Geometry: final body of the model. Coordinates: model frame, mm. A direction names the side the tool comes from. Coordinates: 2 decimals unless noted, no trailing zeros. Order: outer loops, then holes, each group sorted by start corner. A loop starts at its lowest first (then second) coordinate and runs counter-clockwise, first axis right, second up. Notation, with made-up numbers: (43, 36) -> (51, 36) arc R24 cw to (51, 48) -> close; hole circle Ø8 at (55.5, 31.5). An arc over 180 degrees is marked (long way). Use one line per item in the form item = value.
```python
from build123d import *

# Parameters (mm, degrees)
SKETCH1_W           = 33
SKETCH1_H           = 8
SKETCH1_R           = 1.55
BOSS_EXTRUDE1_DEPTH = 4
SKETCH3_W           = 8
SKETCH3_H           = 8
BOSS_EXTRUDE2_DEPTH = 5.5
FILLET1_R           = 2


with BuildPart() as part:
    # Sketch1 → Boss-Extrude1 (new body)
    with BuildSketch(Plane(origin=(0, 0, 0), x_dir=(1, 0, 0), z_dir=(0, 1, 0))):
        with Locations((0.21875, 2.328125)):
            Rectangle(SKETCH1_W, SKETCH1_H)
        with Locations(Location((12.71875, 2.328125, 0), (0, 0, 270))):
            Circle(SKETCH1_R, mode=Mode.SUBTRACT)
    extrude(amount=BOSS_EXTRUDE1_DEPTH)

    # Sketch3 → Boss-Extrude2 (add)
    with BuildSketch(Plane.XZ):
        with Locations((-12.28125, -2.328125)):
            Rectangle(SKETCH3_W, SKETCH3_H)
    extrude(amount=BOSS_EXTRUDE2_DEPTH)

    # Fillet1
    fillet1_edges = [part.edges().sort_by_distance(p)[0] for p in [
        (-16.28125, -5.5, -2.328125),
        (-12.28125, -5.5, -6.328125),
        (-8.28125, -5.5, -2.328125),
        (-12.28125, -5.5, 1.671875),
    ]]
    fillet(fillet1_edges, radius=FILLET1_R)


solid = part.part
```
1) Material intervals for probe 1 along Y at (x, z) = (2.5, -4.5); probe 2 along X at (y, z) = (-1, -2.5); probe 3 along X at (y, z) = (0.25, -3.75), sorted ascending. Write a range as from..to.
Results found:
probe_1 = 0..4
probe_2 = -16.28..-8.28
probe_3 = -16.28..12.1, 13.34..16.72
2) Contact query for a flat-ended pin moving along its axis: P1, Ø1, axis at y = -2.5, z = -1, coming from the +X side. Output: stop coordinate, or through.
Results found:
P1 = -8.28
3) Pull-direction query (Z, two-part tool) for faces 3 (the cylindrical face through (-8.63, -4.63, -2.27)), 4 (the cylindrical face through (11.206, 1.972, -2.664)), 5 (the cylindrical face through (-12.2, -4.6, -6)); classes: released by +Z, released by -Z, zero draft, split by the parting line, or undercut.
Results found:
face_3 = zero draft
face_4 = undercut
face_5 = released by -Z
4) Section A-A, the plane z = -1.75. Output: boundary loops of the cut face in (x, y), and give its area (3 significant figures).
Results found:
outline = (-16.28, -3.5) arc R2 ccw to (-14.28, -5.5) -> (-10.28, -5.5) arc R2 ccw to (-8.28, -3.5) -> (-8.28, 0) -> (11.28, 0) -> (11.28, 4) -> (-16.28, 4) -> close; (14.16, 0) -> (16.72, 0) -> (16.72, 4) -> (14.16, 4) -> close
area = 163 mm2
5) Section B-B, the plane x = 13.5. Output: boundary loops of the cut face in (y, z).
Results found:
outline = (0, -6.33) -> (4, -6.33) -> (4, -3.67) -> (0, -3.67) -> close; (0, -0.99) -> (4, -0.99) -> (4, 1.67) -> (0, 1.67) -> close
6) Access query for faces 1 (the flat face through (-12, -5.5, -2)), 2 (the flat face through (-8.281, -2, -2)). Directions: +Z, -Z, +X, -X, +Y, -Y. A direction counts if a zero-diameter tool reaches every point of the face in a straight line with its end or side. Return the directions, or none.
Results found:
face_1 = +Z, -Z, +X, -X, -Y
face_2 = +Z, -Z, +X, -Y
7) Section D-D, the plane z = -5.5. Output: boundary loops of the cut face in (x, y).
Results found:
outline = (-16.28, -3.5) arc R2 ccw to (-15.45, -5.12) -> (-9.11, -5.12) arc R2 ccw to (-8.28, -3.5) -> (-8.28, 0) -> (16.72, 0) -> (16.72, 4) -> (-16.28, 4) -> close
8) Section C-C, the plane x = -13. Output: boundary loops of the cut face in (y, z), and give its area (3 significant figures).
Results found:
outline = (-5.5, -4.33) arc R2 ccw to (-3.5, -6.33) -> (4, -6.33) -> (4, 1.67) -> (-3.5, 1.67) arc R2 ccw to (-5.5, -0.33) -> close
area = 74.3 mm2
